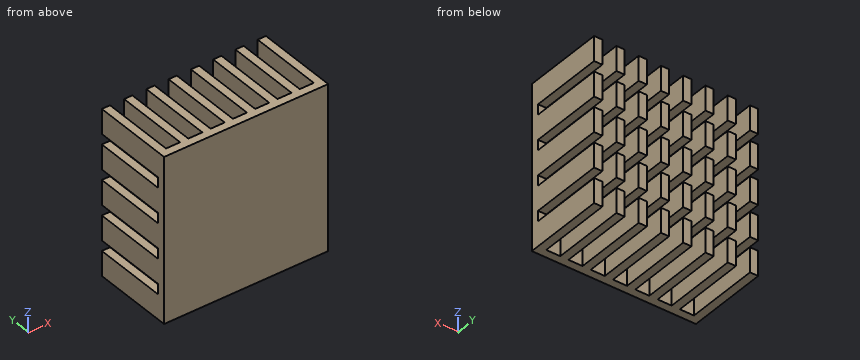
```python
from build123d import *

# Parameters (mm, degrees)
SKETCH1_W           = 20
SKETCH1_H           = 20
BOSS_EXTRUDE1_DEPTH = 1
SKETCH2_W           = 1
SKETCH2_H           = 3
BOSS_EXTRUDE2_DEPTH = 9


with BuildPart() as part:
    # Sketch1 → Boss-Extrude1 (new body)
    with BuildSketch(Plane(origin=(0, 0, 0), x_dir=(1, 0, 0), z_dir=(0, 1, 0))):
        Rectangle(SKETCH1_W, SKETCH1_H)
    extrude(amount=BOSS_EXTRUDE1_DEPTH)

    # Sketch2 → Boss-Extrude2 (add)
    with BuildSketch(Plane(origin=(0, 1, 0), x_dir=(1, 0, 0), z_dir=(0, 1, 0))):
        with Locations((-9.5, 8.5)):
            Rectangle(SKETCH2_W, SKETCH2_H)
        with Locations((-6.78571429, 8.5)):
            Rectangle(SKETCH2_W, SKETCH2_H)
        with Locations((-4.07142858, 8.5)):
            Rectangle(SKETCH2_W, SKETCH2_H)
        with Locations((-1.35714287, 8.5)):
            Rectangle(SKETCH2_W, SKETCH2_H)
        with Locations((1.35714284, 8.5)):
            Rectangle(SKETCH2_W, SKETCH2_H)
        with Locations((4.07142855, 8.5)):
            Rectangle(SKETCH2_W, SKETCH2_H)
        with Locations((6.78571426, 8.5)):
            Rectangle(SKETCH2_W, SKETCH2_H)
        with Locations((9.49999997, 8.5)):
            Rectangle(SKETCH2_W, SKETCH2_H)
        with Locations((6.78571426, 4.25)):
            Rectangle(SKETCH2_W, SKETCH2_H)
        with Locations((4.07142855, 4.25)):
            Rectangle(SKETCH2_W, SKETCH2_H)
        with Locations((1.35714284, 4.25)):
            Rectangle(SKETCH2_W, SKETCH2_H)
        with Locations((-1.35714287, 4.25)):
            Rectangle(SKETCH2_W, SKETCH2_H)
        with Locations((-4.07142858, 4.25)):
            Rectangle(SKETCH2_W, SKETCH2_H)
        with Locations((-9.5, 4.25)):
            Rectangle(SKETCH2_W, SKETCH2_H)
        with Locations((-6.78571429, 0)):
            Rectangle(SKETCH2_W, SKETCH2_H)
        with Locations((-4.07142858, 0)):
            Rectangle(SKETCH2_W, SKETCH2_H)
        with Locations((-1.35714287, 0)):
            Rectangle(SKETCH2_W, SKETCH2_H)
        with Locations((1.35714284, 0)):
            Rectangle(SKETCH2_W, SKETCH2_H)
        with Locations((6.78571426, 0)):
            Rectangle(SKETCH2_W, SKETCH2_H)
        with Locations((9.49999997, 0)):
            Rectangle(SKETCH2_W, SKETCH2_H)
        with Locations((9.49999997, -4.25)):
            Rectangle(SKETCH2_W, SKETCH2_H)
        with Locations((6.78571426, -4.25)):
            Rectangle(SKETCH2_W, SKETCH2_H)
        with Locations((4.07142855, -4.25)):
            Rectangle(SKETCH2_W, SKETCH2_H)
        with Locations((1.35714284, -4.25)):
            Rectangle(SKETCH2_W, SKETCH2_H)
        with Locations((-1.35714287, -4.25)):
            Rectangle(SKETCH2_W, SKETCH2_H)
        with Locations((-4.07142858, -4.25)):
            Rectangle(SKETCH2_W, SKETCH2_H)
        with Locations((-6.78571429, -4.25)):
            Rectangle(SKETCH2_W, SKETCH2_H)
        with Locations((-9.5, -4.25)):
            Rectangle(SKETCH2_W, SKETCH2_H)
        with Locations((-9.5, -8.5)):
            Rectangle(SKETCH2_W, SKETCH2_H)
        with Locations((-6.78571429, -8.5)):
            Rectangle(SKETCH2_W, SKETCH2_H)
        with Locations((-4.07142858, -8.5)):
            Rectangle(SKETCH2_W, SKETCH2_H)
        with Locations((-1.35714287, -8.5)):
            Rectangle(SKETCH2_W, SKETCH2_H)
        with Locations((1.35714284, -8.5)):
            Rectangle(SKETCH2_W, SKETCH2_H)
        with Locations((4.07142855, -8.5)):
            Rectangle(SKETCH2_W, SKETCH2_H)
        with Locations((6.78571426, -8.5)):
            Rectangle(SKETCH2_W, SKETCH2_H)
        with Locations((9.49999997, -8.5)):
            Rectangle(SKETCH2_W, SKETCH2_H)
        with Locations((9.49999997, 4.25)):
            Rectangle(SKETCH2_W, SKETCH2_H)
        with Locations((-6.78571429, 4.25)):
            Rectangle(SKETCH2_W, SKETCH2_H)
        with Locations((-9.5, 0)):
            Rectangle(SKETCH2_W, SKETCH2_H)
        with Locations((4.07142855, 0)):
            Rectangle(SKETCH2_W, SKETCH2_H)
    extrude(amount=BOSS_EXTRUDE2_DEPTH)


solid = part.part
```
Design review of the part built by this model. Coordinates are the model's own, in mm. Give positions to 0.01 mm unless a question says otherwise; leave off trailing zeros. Order: outer loops, then holes, each group sorted by start corner. A loop starts at its lowest first (then second) coordinate and runs counter-clockwise, first axis right, second up. Notation, with made-up numbers: (-28.75, -12) -> (-16.75, -12) arc R26 ccw to (-16.75, 13) -> close; hole circle Ø8 at (-23.75, 24.5). An arc over 180 degrees is marked (long way). Write item = value, one per line. Start each with the question number.
(1) We need section A-A on x = -7. Write out the cut boundary in (y, z).
(2) We need section C-C on y = 4.5. State how many separate pieces and enclosed holes the cut face has, plus the area to 3 significant figures.
(3) We need section D-D on z = -2.25. Write out the cut boundary in (x, y).
(4) To check wall thickness, follow line 1 along Z through (x, y) = (-3.75, 6.5); line 2 along Y through (x, z) = (0.5, -8.75). State the ranges of each line that lie inside material, in increasing order.
Numbers:
q1.outline = (0, -10) -> (10, -10) -> (10, -7) -> (1, -7) -> (1, -5.75) -> (10, -5.75) -> (10, -2.75) -> (1, -2.75) -> (1, -1.5) -> (10, -1.5) -> (10, 1.5) -> (1, 1.5) -> (1, 2.75) -> (10, 2.75) -> (10, 5.75) -> (1, 5.75) -> (1, 7) -> (10, 7) -> (10, 10) -> (0, 10) -> close
q2.separate_pieces = 40
q2.enclosed_holes = 0
q2.area = 120 mm^2
q3.outline = (-10, 0) -> (10, 0) -> (10, 1) -> (-10, 1) -> close
q4.line_1 = -10 to -7, -5.75 to -2.75, -1.5 to 1.5, 2.75 to 5.75, 7 to 10
q4.line_2 = 0 to 1
